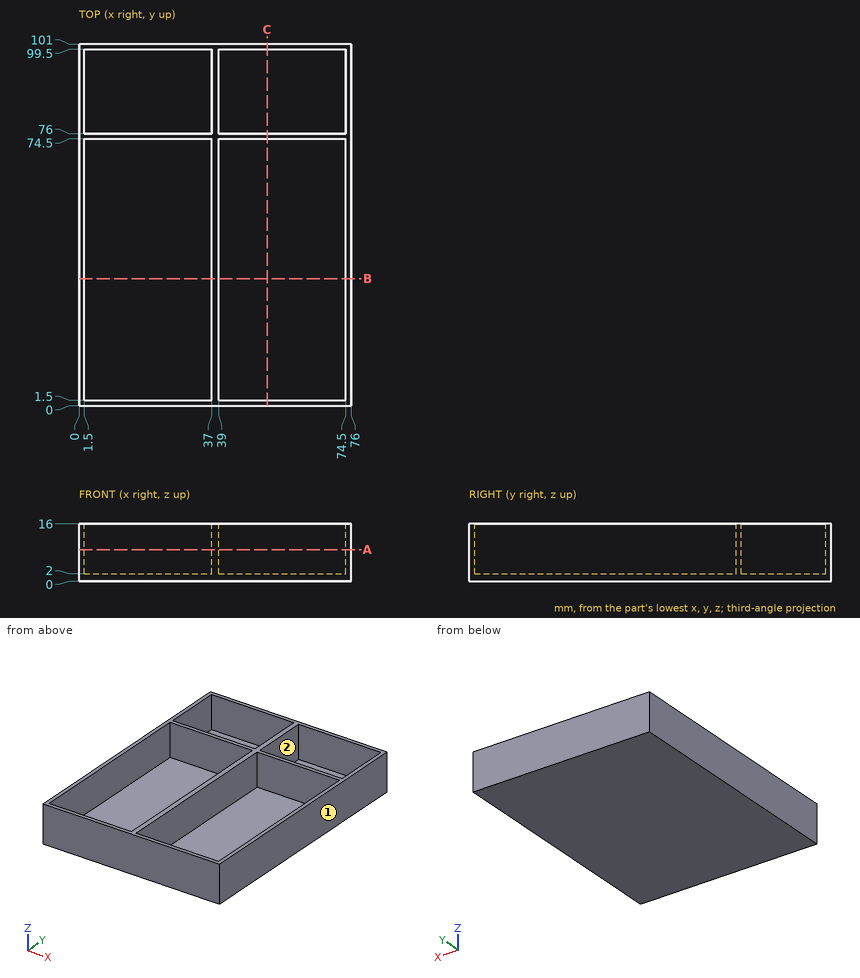
Design review of the part shown in the three views and the two pictorial views. Dimensions are in mm from the part's minimum x, y and z. A direction names the side the tool comes from. Give positions to 0.01 mm unless a question says otherwise; leave off trailing zeros. Order: outer loops, then holes, each group sorted by start corner. A loop starts at its lowest first (then second) coordinate and runs counter-clockwise, first axis right, second up. Notation, with made-up numbers: M 47.25,35.25 L 53.25,35.25 A22 ccw 53.25,56.25 Z; hole C 31.5,6.25 d11. An arc over 180 degrees is marked long. Answer in a Markdown table with one row per item. Add a question column.
(1) Consider section A-A on z = 8.75. State the section outline as (x, y) points.
(2) For pin 1 (18 mm diameter, centred on x = 15.5, y = 43.5, fed in from +Z), flat-tipped, find the tip position at first contact; note if it passes through.
(3) Consider section B-B on y = 35.5. State the section outline as (x, z) points, and give its area (3 significant figures).
(4) Consider section C-C on x = 52.5. State the section outline as (y, z) points, and give its area (3 significant figures).
(5) For the marked faces 1 and 2, list the 3-axis set-ups (+Z, -Z, +X, -X, +Y, -Y) from which the entire face can be reached by the end or side of a thin tool; tool diameter is ignored.
(6) Wall thickness on probe 1 along Y at (x, z) = (6, 13.5); probe 2 along X at (y, z) = (12.5, 8); probe 3 along Z at (x, y) = (24.5, 27.5): over which ranges is each line inside the solid? List them lowest first. Write a range as [from, to].
Evaluation:
| question | item | result |
|---|---|---|
| 1 | outline | M 0,0 L 76,0 L 76,101 L 0,101 Z; hole M 1.5,1.5 L 37,1.5 L 37,74.5 L 1.5,74.5 Z; hole M 1.5,76 L 37,76 L 37,99.5 L 1.5,99.5 Z; hole M 39,1.5 L 74.5,1.5 L 74.5,74.5 L 39,74.5 Z; hole M 39,76 L 74.5,76 L 74.5,99.5 L 39,99.5 Z |
| 2 | pin 1 | stops at z = 2 |
| 3 | outline | M 0,0 L 76,0 L 76,16 L 74.5,16 L 74.5,2 L 39,2 L 39,16 L 37,16 L 37,2 L 1.5,2 L 1.5,16 L 0,16 Z |
| 3 | area | 222 mm^2 |
| 4 | outline | M 0,0 L 101,0 L 101,16 L 99.5,16 L 99.5,2 L 76,2 L 76,16 L 74.5,16 L 74.5,2 L 1.5,2 L 1.5,16 L 0,16 Z |
| 4 | area | 265 mm^2 |
| 5 | face 1 | +Z, -Z, +X, +Y, -Y |
| 5 | face 2 | +Z |
| 6 | probe 1 | y = [0, 1.5], [74.5, 76], [99.5, 101] |
| 6 | probe 2 | x = [0, 1.5], [37, 39], [74.5, 76] |
| 6 | probe 3 | z = [0, 2] |
